For this review, use the dimensioned drawing (mm, ordinates from the lowest corner) and the shaded views. A direction names the side the tool comes from. Round coordinates to 2 decimals unless told otherwise and drop trailing zeros. Order: outer loops, then holes, each group sorted by start corner. A loop starts at its lowest first (then second) coordinate and runs counter-clockwise, first axis right, second up. Notation, with made-up numbers: (11.5, 64.25) -> (67.5, 64.25) arc R6 ccw to (67.5, 69.25) -> close; hole circle Ø5 at (23, 44). An arc over 180 degrees is marked (long way). Use a Markdown table: item, result. Add a question column.
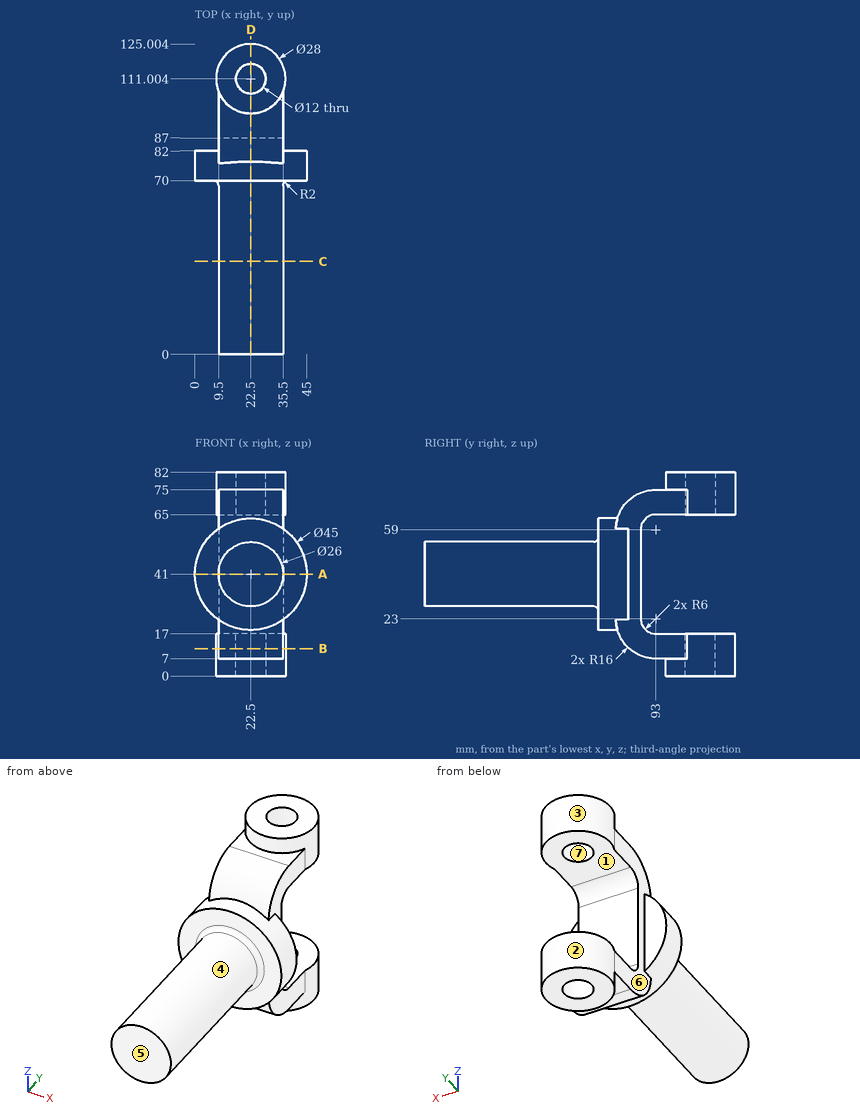
Q1. Wall thickness on line 1 (Y direction, x = 22.5, z = 78.5); line 2 (Z direction, x = 33.5, y = 104); line 3 (Z direction, x = 32, y = 100): over which ranges is each line inside the solid? List them lowest first. Write a range as [from, to].
Q2. Machinability: for the marked faces 1, 2, 3 and 4, which of the approach directions +Z, -Z, +X, -X, +Y, -Y give a long, thin tool a straight path to every point of the face, cutting with its end or side? Answer none if there is none.
Q3. Add section C-C (y = 37.5). Write out the cut boundary in (x, z), then the cut area to 3 significant figures.
Q4. Add section B-B (z = 11). Write out the cut boundary in (x, y), then the cut area to 3 significant figures.
Q5. Add section D-D (x = 22.5). State how many separate pieces and enclosed holes the cut face has, then the cut area to 3 significant figures.
Q6. Mouldability with a two-part tool opening along X and no side actions: class the marked faces 5, 6 and 7 as pulls with the +X half, pulls with the -X half, needs draft (parallel to the pull), parting line crosses it, or undercut.
Q7. Insertion check: pin 1 (14.5 mm diameter, centred on y = 85, z = 41, fed in from -X); pin 2 (8 mm diameter, centred on x = 38.5, z = 59, fed in from -Y); pin 3 (4 mm diameter, centred on x = 20.5, z = 54.5, fed in from +Y); pin 4 (5 mm diameter, centred on x = 40, z = 30.5, fed in from +Y). Each pin has a flat end and moves straight along its axis. Give the tip position at first contact, or say it passes through.
Q8. Add section A-A (z = 41). Write out the cut boundary in (x, y), then the cut area to 3 significant figures.
Report:
| question | item | result |
|---|---|---|
| 1 | line 1 | y = [97, 105], [117, 125] |
| 1 | line 2 | z = [0, 17], [65, 82] |
| 1 | line 3 | z = [7, 17], [65, 75] |
| 2 | face 1 | +X, -X, +Y |
| 2 | face 2 | -Z |
| 2 | face 3 | +Z |
| 2 | face 4 | -Y |
| 3 | outline | circle Ø26 at (22.5, 41) |
| 3 | area | 531 mm² |
| 4 | outline | (9.5, 82.42) -> (35.5, 82.42) -> (35.5, 105.81) arc R14 ccw (long way) to (9.5, 105.81) -> close; hole circle Ø12 at (22.5, 111) |
| 4 | area | 945 mm² |
| 5 | separate pieces | 3 |
| 5 | enclosed holes | 0 |
| 5 | area | 3,470 mm² |
| 6 | face 5 | needs draft |
| 6 | face 6 | pulls with the -X half |
| 6 | face 7 | undercut |
| 7 | pin 1 | stops at x = 0 |
| 7 | pin 2 | stops at y = 70 |
| 7 | pin 3 | stops at y = 87 |
| 7 | pin 4 | stops at y = 82 |
| 8 | outline | (0, 70) -> (7.5, 70) arc R2 cw to (9.5, 68) -> (9.5, 0) -> (35.5, 0) -> (35.5, 68) arc R2 cw to (37.5, 70) -> (45, 70) -> (45, 82) -> (35.5, 82) -> (35.5, 87) -> (9.5, 87) -> (9.5, 82) -> (0, 82) -> close |
| 8 | area | 2,490 mm² |
